from build123d import *

# Parameters (mm, degrees)
EXTRUDE_1_DEPTH     = 24.5
FILLET_1_R          = 25
SKETCH_2_R          = 2
CUT_EXTRUDE_1_DEPTH = 5


with BuildPart() as part:
    # 草图1 → 凸台-拉伸1 (new body)
    with BuildSketch(Plane(origin=(0, 0, 0), x_dir=(1, 0, 0), z_dir=(0, 1, 0))):
        Polygon((-80, 0), (-66.524518745, 40), (65.438851804, 20), (83.060057617, 0), (96.387725214, 0), (90.563245948, 6.610761292), (70.535919799, 29.341698507), (-73.32231493, 51.144450912), (-89.476681383, 3.192571058), (-90.552217169, 0), align=None)
    extrude(amount=EXTRUDE_1_DEPTH)

    # 圆角1
    fillet_1_edges = [part.edges().sort_by_distance(p)[0] for p in [
        (-73.32231493, 12.25, -51.144450912),
        (70.535919799, 12.25, -29.341698507),
        (65.438851804, 12.25, -20),
        (-66.524518745, 12.25, -40),
    ]]
    fillet(fillet_1_edges, radius=FILLET_1_R)

    # 草图2 → 切除-拉伸1 (cut)
    with BuildSketch(Plane.XY):
        with Locations((-85.276108585, 12.25)):
            Circle(SKETCH_2_R)
        with Locations((89.723891415, 12.25)):
            Circle(SKETCH_2_R)
    extrude(amount=-CUT_EXTRUDE_1_DEPTH, mode=Mode.SUBTRACT)


solid = part.part
Input: part model. Units: mm. Frame: model coordinates. A direction names the side the tool comes from. Give positions to 0.01 mm unless a question says otherwise; leave off trailing zeros. Loops run counter-clockwise (first coordinate to the right, second up) from the corner with the lowest first, then second, coordinate; pieces in that order, holes last. Notation, with made-up numbers: M 0.5,36 L 26.5,36 A25 ccw 26.5,62 Z; hole C -20.75,44 d9. An arc over 180 degrees is marked long. Use CSV: the item, a comma, the result in double quotes.
(1) Section A-A, the plane y = 12.25. Return loops of the section in (x, z), plus the area to 3 significant figures.
Outcome:
outline,"M -90.55,0 L -80.02,-31.26 A25 ccw -52.58,-48 L 61.54,-30.71 A25 ccw 76.55,-22.51 L 96.39,0 L 91.72,0 L 91.72,-5 L 87.72,-5 L 87.72,0 L 83.06,0 L 71.45,-13.17 A25 cw 56.44,-21.36 L -45.78,-36.86 A25 cw -73.22,-20.12 L -80,0 L -83.28,0 L -83.28,-5 L -87.28,-5 L -87.28,0 Z"
area,"2,160 mm²"
(2) Pin query (flat end, axial travel): P1, Ø3, axis at x = -44, y = 17, coming from the +Z side; P2, Ø1.2, axis at x = 89.5, y = 12, coming from the +Z side; P3, Ø2, axis at x = 28.5, y = 16, coming from the -Z side. Return the tip coordinate at first contact, or that it passes through.
Outcome:
P1,"stops at z = -36.36"
P2,"stops at z = -5"
P3,"stops at z = -35.86"
(3) Section D-D, the plane x = 10. Return loops of the section in (y, z).
Outcome:
outline,"M 0,-38.52 L 24.5,-38.52 L 24.5,-28.4 L 0,-28.4 Z"
(4) Material intervals for L1, parallel to Z at x = 56, y = 18; L2, parallel to X at y = 7.25, z = -19.5; L3, parallel to Z at x = 83.5, y = 14.5, sorted ascending. Write a range as [from, to].
Outcome:
L1,"z = [-31.54, -21.43]"
L2,"x = [-83.98, -73.43], [62.83, 79.21]"
L3,"z = [-14.63, 0]"
(5) Section B-B, the plane z = -27. Return loops of the section in (x, y).
Outcome:
outline,"M -81.46,0 L -69.63,0 L -69.63,24.5 L -81.46,24.5 Z; M 19.25,0 L 71.34,0 L 71.34,24.5 L 19.25,24.5 Z"
(6) Pull-direction query (Y, two-part tool) for faces 4 (the face through (-4, 0, -31)), 5 (the face through (90, 12, -5)), 6 (the face through (-83.37, 12.85, -2.46)), 7 (the face through (64.56, 12.42, -18.65)); classes: pulls with the +Y half, pulls with the -Y half, needs draft (parallel to the pull), parting line crosses it, or undercut.
Outcome:
face 4,"pulls with the -Y half"
face 5,"undercut"
face 6,"undercut"
face 7,"needs draft"
(7) Set-up query: faces 1 (the face through (-85, 12, -5)), 2 (the face through (-88, 12, 0)), 3 (the face through (77.176, 12.078, -6.679)). Return all of +Z, -Z, +X, -X, +Y, -Y with unobstructed straight access to the full face (end or side cutting, diameter ignored); none if empty.
Outcome:
face 1,"+Z"
face 2,"+Z, +X, -X, +Y, -Y"
face 3,"+Z, +Y, -Y"
(8) Section C-C, the plane z = -11. Return loops of the section in (x, y), plus the area to 3 significant figures.
Outcome:
outline,"M -86.85,0 L -76.29,0 L -76.29,24.5 L -86.85,24.5 Z; M 73.37,0 L 86.7,0 L 86.7,24.5 L 73.37,24.5 Z"
area,"585 mm²"
